from build123d import *

# Parameters (mm, degrees)
F1_DEPTH = 25.4
F2_R     = 12.7
F3_DEPTH = 61.57864
F4_R     = 3.175
F5_DEPTH = 12.7


with BuildPart() as f1:
    # F0 (on Front) → F1 (new body)
    with BuildSketch(Plane.XZ):
        with BuildLine():
            Line((-7.068471, 25.4), (-7.068471, 0))
            Line((-7.068471, 0), (31.031529, 0))
            Line((31.031529, 0), (31.031529, 25.4))
            ThreePointArc((31.031529, 25.4), (25.451913, 38.870384), (11.981529, 44.45))
            ThreePointArc((11.981529, 44.45), (-1.488855, 38.870384), (-7.068471, 25.4))
        make_face()
    extrude(amount=F1_DEPTH)

    # F2 (on face) → F3 (cut)
    with BuildSketch(Plane.XZ.offset(25.4)):
        with Locations((11.981529, 25.4)):
            Circle(F2_R)
    extrude(amount=-F3_DEPTH, mode=Mode.SUBTRACT)

    # F4 (on face) → F5 (cut)
    with BuildSketch(Plane(origin=(0, 0, 0), x_dir=(1, 0, 0), z_dir=(0, 0, -1))):
        with Locations((-0.718471, 12.7)):
            Circle(F4_R)
        with Locations((24.681529, 12.7)):
            Circle(F4_R)
    extrude(amount=-F5_DEPTH, mode=Mode.SUBTRACT)


solid = f1.part
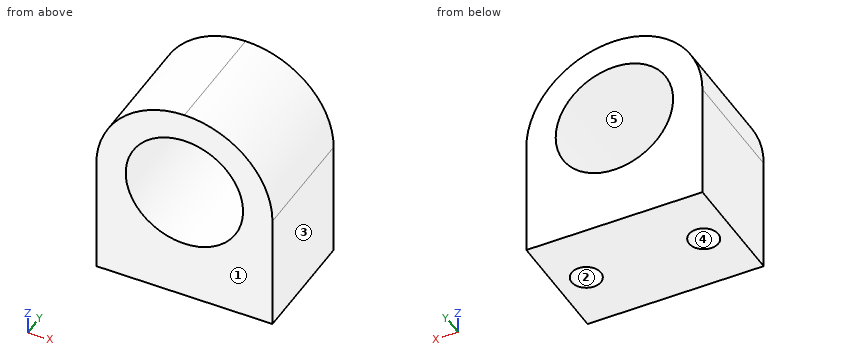
Part model, mm, in its own coordinate system. Face numbers are marked on the shaded views. A direction names the side the tool comes from. Round coordinates to 2 decimals unless told otherwise and drop trailing zeros. Order: outer loops, then holes, each group sorted by start corner. A loop starts at its lowest first (then second) coordinate and runs counter-clockwise, first axis right, second up. Notation, with made-up numbers: (-8.5, 78.25) -> (46.5, 78.25) arc R23 cw to (46.5, 97.25) -> close; hole circle Ø9 at (38, 65.25). An arc over 180 degrees is marked (long way). Put each result on its own line as item: value.
Q1. Wall check: line 1 (X direction, y = -12.7, z = 3.5); line 2 (X direction, y = -11.5, z = 8.5); line 3 (Z direction, x = 4, y = -15.5). Give the ranges that are in metal, low to high. Write a range as [from, to].
From the geometry:
line 1: x = [-7.07, -3.89], [2.46, 21.51], [27.86, 31.03]
line 2: x = [-7.07, -3.66], [2.22, 21.74], [27.62, 31.03]
line 3: z = [0, 15.52], [35.28, 42.7]
Q2. Pull direction Y, two halves, no side cores. Call the marked faces 1, 2 and 3: pulls with the +Y half, pulls with the -Y half, needs draft (parallel to the pull), parting line crosses it, or undercut.
From the geometry:
face 1: pulls with the -Y half
face 2: undercut
face 3: needs draft
Q3. Tool access for the marked faces 4 and 5: list every direction of +Z, -Z, +X, -X, +Y, -Y with a clear straight run to the whole face (end or side of a thin tool).
From the geometry:
face 4: -Z
face 5: +Y, -Y
Q4. Pin check, flat tips, straight feed: pin 1 Ø3 at (y, z) = (-9.5, 28.5) entering from -X; pin 2 Ø5 at (y, z) = (-14, 32.5) entering from -X; pin 3 Ø4 at (x, y) = (24.68, -12.7) entering from +Z. Stop position of each tip, or through.
From the geometry:
pin 1: stops at x = -7
pin 2: stops at x = -6.5
pin 3: stops at z = 41.16
Q5. Band-saw the part on B-B (x = 1). Give the cut face in (y, z), and give its area (3 significant figures).
From the geometry:
outline: (-25.4, 0) -> (-15.37, 0) -> (-15.37, 12.7) -> (-10.03, 12.7) -> (-10.03, 0) -> (0, 0) -> (0, 19.02) -> (-25.4, 19.02) -> close; (-25.4, 31.78) -> (0, 31.78) -> (0, 40.97) -> (-25.4, 40.97) -> close
area: 649 mm2
Q6. Band-saw the part on C-C (z = 17.5). Give the cut face in (x, y), and give its area (3 significant figures).
From the geometry:
outline: (-7.07, -25.4) -> (2.04, -25.4) -> (2.04, 0) -> (-7.07, 0) -> close; (21.93, -25.4) -> (31.03, -25.4) -> (31.03, 0) -> (21.93, 0) -> close
area: 463 mm2
Q7. Band-saw the part on D-D (y = -12.7). Give the cut face in (x, z), and give its area (3 significant figures).
From the geometry:
outline: (-7.07, 0) -> (-3.89, 0) -> (-3.89, 12.7) -> (2.46, 12.7) -> (2.46, 0) -> (21.51, 0) -> (21.51, 12.7) -> (27.86, 12.7) -> (27.86, 0) -> (31.03, 0) -> (31.03, 25.4) arc R19.05 ccw to (11.98, 44.45) arc R19.05 ccw to (-7.07, 25.4) -> close; hole circle Ø25.4 at (11.98, 25.4)
area: 870 mm2
Q8. Band-saw the part on A-A (y = -3). Give the cut face in (x, z), and give its area (3 significant figures).
From the geometry:
outline: (-7.07, 0) -> (31.03, 0) -> (31.03, 25.4) arc R19.05 ccw to (11.98, 44.45) arc R19.05 ccw to (-7.07, 25.4) -> close; hole circle Ø25.4 at (11.98, 25.4)
area: 1,030 mm2
